The model under review builds one solid part; all positions refer to its coordinate system, in mm. Face numbers are marked on the shaded views. A direction names the side the tool comes from. Coordinates: 2 decimals unless noted, no trailing zeros. Order: outer loops, then holes, each group sorted by start corner. A loop starts at its lowest first (then second) coordinate and runs counter-clockwise, first axis right, second up. Notation, with made-up numbers: (81.5, -39) -> (88.5, -39) arc R11 ccw to (88.5, -35) -> close; hole circle Ø10 at (-19.5, -1). An arc over 180 degrees is marked (long way). Use one line per item in the form item = value. Start each with the question number.
(1) Wall thickness on line 1 along Z through (x, y) = (19.5, 0.6); line 2 along X through (y, z) = (23.75, -11.5) (3 decimals); line 3 along X through (y, z) = (1.6, 31): over which ranges is each line inside the solid? List them lowest first.
(2) Take a section at D-D (y = 23.5). State the section outline as (x, z) points (3 decimals), then the cut area to 3 significant figures.
(3) Take a section at A-A (z = -31). State the section outline as (x, y) points (3 decimals), then the cut area to 3 significant figures.
(4) Take a section at B-B (y = 10.75). State the section outline as (x, z) points (3 decimals).
(5) Insertion check: pin 1 Ø4 at (x, z) = (-19.5, 37.6) entering from -Y; pin 2 Ø1.5 at (x, z) = (-11, -18.5) entering from +Y; pin 3 Ø4 at (x, z) = (19.5, 31) entering from +Y. Each pin has a flat end and moves straight along its axis. Give the tip position at first contact, or say it passes through.
(6) Take a section at C-C (x = 19.5). State the section outline as (y, z) points.
(7) For the marked faces 1 and 2, list the 3-axis set-ups (+Z, -Z, +X, -X, +Y, -Y) from which the entire face can be reached by the end or side of a thin tool; tool diameter is ignored.
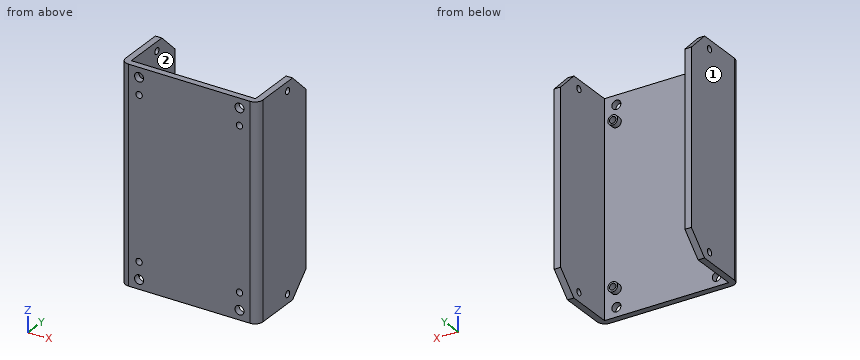
```python
from build123d import *

# Parameters (mm, degrees)
EXTRUDE_1_DEPTH          = 41.25
CUT_EXTRUDE_1_DEPTH      = 58.02151458
CUT_EXTRUDE_1_DEPTH_BACK = 58.02151458
SKETCH_4_R               = 1.75
CUT_EXTRUDE_2_DEPTH      = 10
HOLE_WIZARD_M31_REACH    = 75.336
HOLE_WIZARD_M31_BORE_R   = 1.25
HOLE_WIZARD_M32_D        = 2.5
SKETCH_10_R              = 1.9
EXTRUDE_2_DEPTH          = 2.2
HOLE_WIZARD_M33_D        = 2.5


with BuildPart() as part:
    # Эскиз1 → Бобышка-Вытянуть1 (new, symmetric)
    with BuildSketch(Plane.XY):
        with BuildLine():
            Line((-26.625, 29), (-26.625, 3))
            ThreePointArc((-26.625, 3), (-25.746320344, 0.878679656), (-23.625, 0))
            Line((-23.625, 0), (23.625, 0))
            ThreePointArc((23.625, 0), (25.746320344, 0.878679656), (26.625, 3))
            Line((26.625, 3), (26.625, 29))
            Line((26.625, 29), (24.125, 29))
            Line((24.125, 29), (24.125, 2.5))
            Line((24.125, 2.5), (-24.125, 2.5))
            Line((-24.125, 2.5), (-24.125, 29))
            Line((-24.125, 29), (-26.625, 29))
        make_face()
    extrude(amount=EXTRUDE_1_DEPTH, both=True)

    # Эскиз3 → Вырез-Вытянуть1 (cut, two sides: drawn at the far end of the back side and taken through both)
    with BuildSketch(Plane(origin=(0, 0, 0), x_dir=(0, 0, -1), z_dir=(1, 0, 0)).offset(-CUT_EXTRUDE_1_DEPTH_BACK)):
        Polygon((41.25, 21), (41.25, 29), (33.5, 29), align=None)
        Polygon((-41.25, 21), (-41.25, 29), (-33.5, 29), align=None)
    extrude(amount=CUT_EXTRUDE_1_DEPTH + CUT_EXTRUDE_1_DEPTH_BACK, mode=Mode.SUBTRACT)

    # Эскиз4 → Вырез-Вытянуть2 (cut)
    with BuildSketch(Plane.XZ):
        with Locations((-19.5, -37.6)):
            Circle(SKETCH_4_R)
        with Locations((-19.5, 37.6)):
            Circle(SKETCH_4_R)
        with Locations((19.5, 37.6)):
            Circle(SKETCH_4_R)
        with Locations((19.5, -37.6)):
            Circle(SKETCH_4_R)
    extrude(amount=-CUT_EXTRUDE_2_DEPTH, mode=Mode.SUBTRACT)

    # Отверстие обработанное метчиком M31 bore → Отверстие обработанное метчиком M31 (cut, up to next)
    with BuildSketch(Plane(origin=(26.625, 0, 0), x_dir=(0, 0, -1), z_dir=(1, 0, 0)), mode=Mode.PRIVATE) as hole_wizard_m31_sk1:
        with Locations((37.75, 18)):
            Circle(HOLE_WIZARD_M31_BORE_R)
    hole_wizard_m31_tool1 = extrude(hole_wizard_m31_sk1.sketch, amount=-HOLE_WIZARD_M31_REACH, mode=Mode.PRIVATE) & part.part
    # Отверстие обработанное метчиком M31 bore → Отверстие обработанное метчиком M31 (cut, up to next)
    with BuildSketch(Plane(origin=(26.625, 0, 0), x_dir=(0, 0, -1), z_dir=(1, 0, 0)), mode=Mode.PRIVATE) as hole_wizard_m31_sk2:
        with Locations((-37.75, 18)):
            Circle(HOLE_WIZARD_M31_BORE_R)
    hole_wizard_m31_tool2 = extrude(hole_wizard_m31_sk2.sketch, amount=-HOLE_WIZARD_M31_REACH, mode=Mode.PRIVATE) & part.part
    add(hole_wizard_m31_tool1.solids().sort_by_distance((26.625, 18, -37.75))[0], mode=Mode.SUBTRACT)
    add(hole_wizard_m31_tool2.solids().sort_by_distance((26.625, 18, 37.75))[0], mode=Mode.SUBTRACT)

    # Отверстие обработанное метчиком M32 (through all)
    with Locations(Plane.ZY.offset(26.625)):
        with Locations((-37.75, 18), (37.75, 18)):
            Hole(HOLE_WIZARD_M32_D / 2)

    # Эскиз10 → Бобышка-Вытянуть2 (add)
    with BuildSketch(Plane(origin=(0, 2.5, 0), x_dir=(1, 0, 0), z_dir=(0, 1, 0))):
        with Locations(Location((19.5, 31, 0), (0, 0, 90))):
            Circle(SKETCH_10_R)
        with Locations(Location((19.5, -31, 0), (0, 0, 90))):
            Circle(SKETCH_10_R)
        with Locations(Location((-19.5, -31, 0), (0, 0, 90))):
            Circle(SKETCH_10_R)
        with Locations(Location((-19.5, 31, 0), (0, 0, 90))):
            Circle(SKETCH_10_R)
    extrude(amount=EXTRUDE_2_DEPTH)

    # Отверстие обработанное метчиком M33 (through all)
    with Locations(Plane(origin=(0, 4.7, 0), x_dir=(1, 0, 0), z_dir=(0, 1, 0))):
        with Locations((19.5, 31), (-19.5, 31), (19.5, -31), (-19.5, -31)):
            Hole(HOLE_WIZARD_M33_D / 2)


solid = part.part
```
Findings:
q1.line_1 = -41.25 to -39.35, -35.85 to -32.25, -29.75 to 29.75, 32.25 to 35.85, 39.35 to 41.25
q1.line_2 = -26.625 to -24.125, 24.125 to 26.625
q1.line_3 = -26.28 to -20.75, -18.25 to 18.25, 20.75 to 26.28
q2.outline = (-26.625, -38.828) -> (-24.125, -38.828) -> (-24.125, 38.828) -> (-26.625, 38.828) -> close; (24.125, -38.828) -> (26.625, -38.828) -> (26.625, 38.828) -> (24.125, 38.828) -> close
q2.area = 388 mm²
q3.outline = (-26.625, 3) arc R3 ccw to (-23.625, 0) -> (-20.75, 0) -> (-20.75, 4.7) -> (-21.4, 4.7) -> (-21.4, 2.5) -> (-24.125, 2.5) -> (-24.125, 29) -> (-26.625, 29) -> close; (-18.25, 0) -> (18.25, 0) -> (18.25, 4.7) -> (17.6, 4.7) -> (17.6, 2.5) -> (-17.6, 2.5) -> (-17.6, 4.7) -> (-18.25, 4.7) -> close; (20.75, 0) -> (23.625, 0) arc R3 ccw to (26.625, 3) -> (26.625, 29) -> (24.125, 29) -> (24.125, 2.5) -> (21.4, 2.5) -> (21.4, 4.7) -> (20.75, 4.7) -> close
q3.area = 255 mm²
q4.outline = (-26.625, -41.25) -> (-24.125, -41.25) -> (-24.125, 41.25) -> (-26.625, 41.25) -> close; (24.125, -41.25) -> (26.625, -41.25) -> (26.625, 41.25) -> (24.125, 41.25) -> close
q5.pin_1 = 0
q5.pin_2 = 2.5
q5.pin_3 = 4.7
q6.outline = (0, -41.25) -> (2.5, -41.25) -> (2.5, -39.35) -> (0, -39.35) -> close; (0, -35.85) -> (2.5, -35.85) -> (2.5, -32.9) -> (4.7, -32.9) -> (4.7, -32.25) -> (0, -32.25) -> close; (0, -29.75) -> (4.7, -29.75) -> (4.7, -29.1) -> (2.5, -29.1) -> (2.5, 29.1) -> (4.7, 29.1) -> (4.7, 29.75) -> (0, 29.75) -> close; (0, 32.25) -> (4.7, 32.25) -> (4.7, 32.9) -> (2.5, 32.9) -> (2.5, 35.85) -> (0, 35.85) -> close; (0, 39.35) -> (2.5, 39.35) -> (2.5, 41.25) -> (0, 41.25) -> close
q7.face_1 = +Z, -Z, -X, +Y, -Y
q7.face_2 = +Z, -Z, +Y
